Autodesk Inventor part; units mm, degrees
ref_plane "YZ Plane" through (0, 0, 0) normal (1, 0, 0) x (0, 1, 0)
ref_plane "XZ Plane" through (0, 0, 0) normal (0, 1, 0) x (-1, 0, 0)
ref_plane "XY Plane" through (0, 0, 0) normal (0, 0, 1) x (1, 0, 0)
sketch "Sketch1" plane through (0, 0, 0) normal (1, 0, 0) x (0, 1, 0)
  line L0 (0, 0) -> (0, -12)
  line L1 (0, -12) -> (3, -12)
  line L2 (3, -12) -> (1.5, -10.5)
  line L3 (1.5, -10.5) -> (1.5, 0)
  line L4 (1.5, 0) -> (0, 0)
  dimension "d0" = 6
  dimension "d1" = 12
  dimension "d2" = 45
  dimension "d3" = 3
revolve "Revolution1" add sketch "Sketch1" angle 360 about axis through (0, 0, 0) along (0, 0, -1)
chamfer "Chamfer1" distance 0.2 angle 45 1 edges at (0, -1.5, 0)
thread "Thread1"
sketch "Sketch2" plane through (0, 0, -12) normal (0, 0, -1) x (-1, 0, 0)
  circle A0 centre (0, 0) radius 1.3
  line L0 (1.1547, 0) -> (0.5774, -1)
  line L1 (0.5774, -1) -> (-0.5774, -1)
  line L2 (-0.5774, -1) -> (-1.1547, 0)
  line L3 (-1.1547, 0) -> (-0.5774, 1)
  line L4 (-0.5774, 1) -> (0.5774, 1)
  line L5 (0.5774, 1) -> (1.1547, 0)
  dimension "d10" = 2
extrude "Extrusion1" cut sketch "Sketch2" against normal blind 1.2 contours L0 L1 L2 L3 L4 L5
properties part number "M3 x 10mm FHCS"
Work out the finished part from the listing and answer in its coordinate system (mm). A direction names the side the tool comes from. Coordinates: 2 decimals unless noted, no trailing zeros. Write each loop counter-clockwise with the first axis right and the second up, starting at its lowest first coordinate (ties: lowest second). Pieces come first, ordered by that corner, then holes.
Q1. Determine the mould class of faces 3 (the face through (-0.86, 0.51, -11.41)), 4 (the face through (-0.07, -1.5, -5.28)), 5 (the face through (0, 1.3, -12)) for opening direction Y: released by +Y, released by -Y, zero draft, split by the parting line, or undercut.
Q2. A cutting plane is placed at A-A, the plane z = -11. Give the vertices of the cut face in (x, y).
Q3. A cutting plane is placed at C-C, the plane z = -8.5. Give the vertices of the cut face in (x, y), then the cut area to 3 significant figures.
Q4. Find the intervals of material crossed by line 1 (Z direction, x = 0.05, y = -0.7); line 2 (Y direction, x = 0.1, z = -6); line 3 (Y direction, x = 1.1, z = -6.75), in increasing order.
Q5. Which of the six approach directions +Z, -Z, +X, -X, +Y, -Y give full straight-line access (tool end or side, diameter ignored) to faces 1 (the face through (-2, 0, -11)), 2 (the face through (0, 1, -11))?
Q6. Each of these flat-tipped pins is pushed along its axis until it touches: pin 1 Ø0.9 at (x, z) = (-0.5, -11.5) entering from -Y; pin 2 Ø3 at (x, z) = (1, -7.5) entering from -Y; pin 3 Ø3 at (y, z) = (2, -8.5) entering from +X. Where does it stop, or does it pass through?
Q7. A cutting plane is placed at B-B, the plane x = 0. Give the vertices of the cut face in (y, z).
Findings below:
1. face 3: undercut
1. face 4: split by the parting line
1. face 5: zero draft
2. outline: circle Ø4 at (0, 0); hole (-1.15, 0) - (-0.58, -1) - (0.58, -1) - (1.15, 0) - (0.58, 1) - (-0.58, 1) - close
3. outline: circle Ø3 at (0, 0)
3. area: 7.07 mm2
4. line 1: z = -10.8 to 0
4. line 2: y = -1.5 to 1.5
4. line 3: y = -1.02 to 1.02
5. face 1: +Z
5. face 2: -Z
6. pin 1: stops at y = -2.91
6. pin 2: stops at y = -1.5
6. pin 3: stops at x = 1.41
7. outline: (-3, -12) - (-1, -12) - (-1, -10.8) - (1, -10.8) - (1, -12) - (3, -12) - (1.5, -10.5) - (1.5, -0.2) - (1.3, 0) - (-1.3, 0) - (-1.5, -0.2) - (-1.5, -10.5) - close
